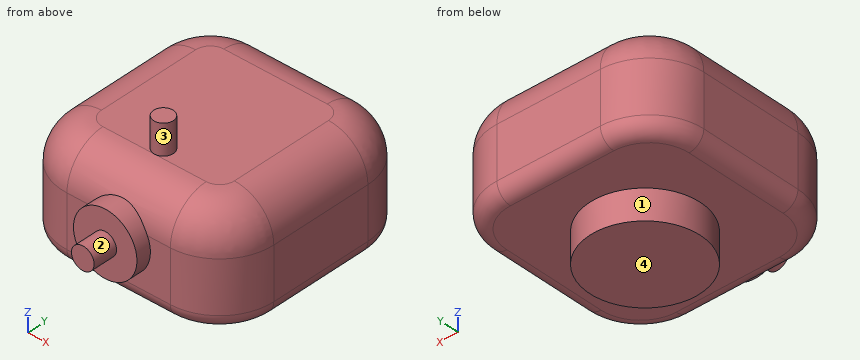
Autodesk Inventor part; units mm, degrees
ref_plane "YZ Plane" through (0, 0, 0) normal (1, 0, 0) x (0, 1, 0)
ref_plane "XZ Plane" through (0, 0, 0) normal (0, 1, 0) x (-1, 0, 0)
ref_plane "XY Plane" through (0, 0, 0) normal (0, 0, 1) x (1, 0, 0)
sketch "스케치1" plane through (0, 0, 0) normal (0, 0, 1) x (1, 0, 0)
  line L0 (21.5, -21.5) -> (-21.5, -21.5)
  line L1 (-21.5, -21.5) -> (-21.5, 21.5)
  line L2 (-21.5, 21.5) -> (21.5, 21.5)
  line L3 (21.5, 21.5) -> (21.5, -21.5)
  line L4 (21.5, -21.5) -> (-21.5, 21.5) construction
  line L5 (-21.5, -21.5) -> (21.5, 21.5) construction
  point P0 (0, 0)
  dimension "d0" = 43
  dimension "d1" = 43
extrude "돌출1" add sketch "스케치1" along normal blind 21.5
sketch "스케치2" plane through (0, 0, 0) normal (0, 0, -1) x (-1, 0, 0)
  circle A0 centre (0, 0) radius 11.2
  dimension "d4" = 22.4
extrude "돌출2" add sketch "스케치2" along normal blind 6.1
sketch "스케치3" plane through (0, 0, 21.5) normal (0, 0, 1) x (1, 0, 0)
  line L0 (-21.5, -21.5) -> (21.5, -21.5)
  circle A0 centre (0, -11.5) radius 2
  point P0 (0, 0)
  dimension "d7" = 4
  dimension "d8" = 10
extrude "돌출3" add sketch "스케치3" along normal blind 6.1
sketch "스케치4" plane through (-21.5, -21.5, 0) normal (0, -1, 0) x (1, 0, 0)
  line L0 (43, 0) -> (43, 21.5)
  line L1 (0, 21.5) -> (43, 21.5)
  line L2 (0, 0) -> (0, 21.5)
  line L3 (43, 10.75) -> (0, 10.75) construction
  line L4 (21.5, 0) -> (21.5, 21.5) construction
  circle A0 centre (21.5, 10.75) radius 6.45
  circle A1 centre (21.5, 10.75) radius 2.3
  dimension "d11" = 12.9
  dimension "d12" = 4.6
extrude "돌출4" add sketch "스케치4" along normal blind 8 contours A1
extrude "돌출5" add sketch "스케치4" along normal blind 3
fillet "모깎기1" radius 11 4 edges at (-21.5, -21.5, 10.75) (21.5, -21.5, 10.75) (-21.5, 21.5, 10.75) (21.5, 21.5, 10.75)
fillet "모깎기2" radius 8 8 edges at (0, -21.5, 21.5) (-18.2782, -18.2782, 21.5) (-21.5, 0, 21.5) (-18.2782, 18.2782, 21.5) (0, 21.5, 21.5) (18.2782, 18.2782, 21.5) (21.5, 0, 21.5) (18.2782, -18.2782, 21.5)
fillet "모깎기3" radius 3 8 edges at (21.5, 0, 0) (18.2782, 18.2782, 0) (0, 21.5, 0) (-18.2782, 18.2782, 0) (-21.5, 0, 0) (-18.2782, -18.2782, 0) (0, -21.5, 0) (18.2782, -18.2782, 0)
equation "\"d1\" = d0"
properties part number "camera" material "고무, 검은색"
Source: CAD feature listing. Evaluate the final solid. Frame: model axes, mm. Face numbers are marked on the shaded views. A direction names the side the tool comes from. Give positions to 0.01 mm unless a question says otherwise; leave off trailing zeros. Write each loop counter-clockwise with the first axis right and the second up, starting at its lowest first coordinate (ties: lowest second). Pieces come first, ordered by that corner, then holes. Notation, with made-up numbers: (-22, 88) - (29, 88) arc R13 ccw to (29, 100) - close; hole circle Ø1 at (24, 62). An arc over 180 degrees is marked (long way). One line per item, written item: value. Start each with the question number.
Q1. Section query D-D, the plane z = -1. Return the cut outline in (x, y), then the cut area to 3 significant figures.
Q2. Material intervals for probe 1 along Z at (x, y) = (10.5, 1); probe 2 along Y at (x, z) = (-7, 13.5); probe 3 along Y at (x, z) = (-3.5, 12), sorted ascending. Write a range as from..to.
Q3. Section query C-C, the plane x = 9.5. Return the cut outline in (y, z), then the cut area to 3 significant figures.
Q4. Set-up query: the marked faces 1, 2, 3 and 4. Return all of +Z, -Z, +X, -X, +Y, -Y with unobstructed straight access to the full face (end or side cutting, diameter ignored); none if empty.
Q5. First-contact query: pin 1 Ø12 at (x, z) = (12.5, 1) entering from -Y; pin 2 Ø4 at (y, z) = (-12, -1.5) entering from +X; pin 3 Ø13.5 at (x, y) = (-6, -1) entering from +Z; pin 4 Ø14 at (x, z) = (2.5, 12) entering from -Y. Flat tips, straight axial feed; report the tip coordinate or a pass-through.
Q6. Section query B-B, the plane y = 0. Return the cut outline in (x, z), then the cut area to 3 significant figures.
Q7. Section query A-A, the plane z = 10.75. Return the cut outline in (x, y), then the cut area to 3 significant figures.
Answer:
1. outline: circle Ø22.4 at (0, 0)
1. area: 394 mm2
2. probe 1: z = -6.1..21.5
2. probe 2: y = -21.5..21.5
2. probe 3: y = -24.5..21.5
3. outline: (-21.5, 3) arc R3 ccw to (-18.5, 0) - (-5.93, 0) - (-5.93, -6.1) - (5.93, -6.1) - (5.93, 0) - (18.5, 0) arc R3 ccw to (21.5, 3) - (21.5, 13.5) arc R8 ccw to (13.5, 21.5) - (-13.5, 21.5) arc R8 ccw to (-21.5, 13.5) - close
3. area: 966 mm2
4. face 1: -Z
4. face 2: -Y
4. face 3: +Z
4. face 4: -Z, +X, -X, +Y, -Y
5. pin 1: stops at y = -21.5
5. pin 2: stops at x = 20.06
5. pin 3: stops at z = 21.5
5. pin 4: stops at y = -29.5
6. outline: (-21.5, 3) arc R3 ccw to (-18.5, 0) - (-11.2, 0) - (-11.2, -6.1) - (11.2, -6.1) - (11.2, 0) - (18.5, 0) arc R3 ccw to (21.5, 3) - (21.5, 13.5) arc R8 ccw to (13.5, 21.5) - (-13.5, 21.5) arc R8 ccw to (-21.5, 13.5) - close
6. area: 1,030 mm2
7. outline: (-21.5, -10.5) arc R11 ccw to (-10.5, -21.5) - (-6.45, -21.5) - (-6.45, -24.5) - (-2.3, -24.5) - (-2.3, -29.5) - (2.3, -29.5) - (2.3, -24.5) - (6.45, -24.5) - (6.45, -21.5) - (10.5, -21.5) arc R11 ccw to (21.5, -10.5) - (21.5, 10.5) arc R11 ccw to (10.5, 21.5) - (-10.5, 21.5) arc R11 ccw to (-21.5, 10.5) - close
7. area: 1,810 mm2
